Geometry check sheet. Reference: drawing and pictorial views, mm from the part's lowest x, y, z. A direction names the side the tool comes from. Give positions to 0.01 mm unless a question says otherwise; leave off trailing zeros. Write each loop counter-clockwise with the first axis right and the second up, starting at its lowest first coordinate (ties: lowest second). Pieces come first, ordered by that corner, then holes. Notation, with made-up numbers: M 4.25,-36.5 L 8.25,-36.5 A9 ccw 8.25,-24.5 Z; hole C 76,55.25 d9. An arc over 180 degrees is marked long. One line per item, written item: value. Start each with the question number.
1. Cross-section at C-C on z = 0.75. Record the cut outline in (x, y) (1 decimal).
2. Cross-section at A-A on y = 14.55. Record the cut outline in (x, z).
3. Tool access check on the marked faces 1, 2 and 3. Record the directions out of +Z, -Z, +X, -X, +Y, -Y that give a thin tool (end or side, any length) a straight path to the whole face; none if there is none.
4. Gauge pin test, flat ends, axial feed: pin 1 (1 mm diameter, centred on y = 12.5, z = 3.5, fed in from -X); pin 2 (1 mm diameter, centred on x = 10.5, z = 3.5, fed in from -Y); pin 3 (2 mm diameter, centred on x = 14.5, z = 3.5, fed in from +Y). Record the tip position at first contact, or that the pin passes through.
5. Release check for a two-part mould opening along X. For the marked faces 4, 5 and 6 record: pulls with the +X half, pulls with the -X half, needs draft (parallel to the pull), parting line crosses it, or undercut.
6. Scan lines: line 1 (Y direction, x = 22, z = 0.7); line 2 (X direction, y = 17, z = 2.25); line 3 (Z direction, x = 9, y = 16.5). Record each from-to range of solid material in increasing order.
7. Cross-section at D-D on x = 12.5. Record the cut outline in (y, z).
8. Cross-section at B-B on x = 23. Record the cut outline in (y, z).
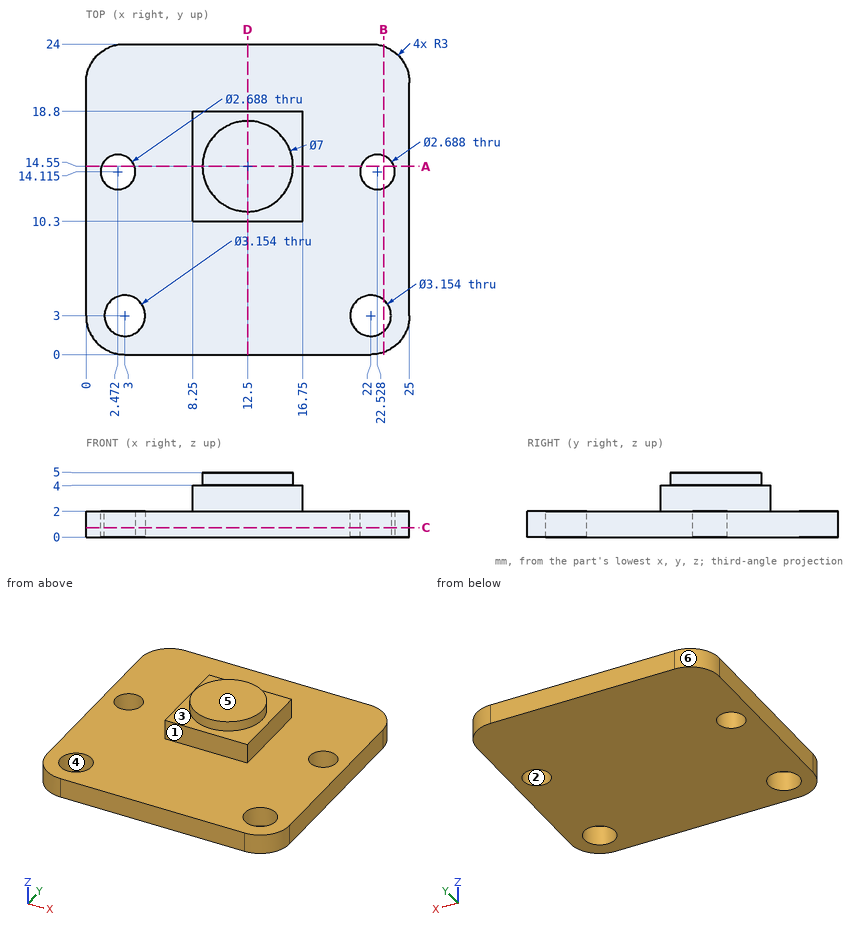
Report:
1. outline: M 0,3 A3 ccw 3,0 L 22,0 A3 ccw 25,3 L 25,21 A3 ccw 22,24 L 3,24 A3 ccw 0,21 Z; hole C 2.5,14.1 d2.7; hole C 3,3 d3.2; hole C 22,3 d3.2; hole C 22.5,14.1 d2.7
2. outline: M 0,0 L 1.2,0 L 1.2,2 L 0,2 Z; M 3.74,0 L 21.26,0 L 21.26,2 L 16.75,2 L 16.75,4 L 16,4 L 16,5 L 9,5 L 9,4 L 8.25,4 L 8.25,2 L 3.74,2 Z; M 23.8,0 L 25,0 L 25,2 L 23.8,2 Z
3. face 1: +Z, +X, -X, -Y
3. face 2: +Z, -Z
3. face 3: +Z
4. pin 1: stops at x = 8.25
4. pin 2: stops at y = 10.3
4. pin 3: stops at y = 18.8
5. face 4: undercut
5. face 5: needs draft
5. face 6: pulls with the -X half
6. line 1: y = 0 to 1.42, 4.58 to 12.88, 15.35 to 24
6. line 2: x = 8.25 to 16.75
6. line 3: z = 0 to 4
7. outline: M 0,0 L 24,0 L 24,2 L 18.8,2 L 18.8,4 L 18.05,4 L 18.05,5 L 11.05,5 L 11.05,4 L 10.3,4 L 10.3,2 L 0,2 Z
8. outline: M 0.17,0 L 1.78,0 L 1.78,2 L 0.17,2 Z; M 4.22,0 L 12.86,0 L 12.86,2 L 4.22,2 Z; M 15.37,0 L 23.83,0 L 23.83,2 L 15.37,2 Z
